```python
from build123d import *


with BuildPart() as part:
    # Sketch1 → Base-Revolve (revolve)
    with BuildSketch(Plane.XY, mode=Mode.PRIVATE) as base_revolve_sk:
        with BuildLine():
            Line((0, 8), (0, 6.794144144))
            ThreePointArc((0, 6.794144144), (0.796034843, 5.848666431), (-0.1025, 5))
            Line((-0.1025, 5), (-40.113248654, 5))
            Line((-40.113248654, 5), (-43, 10))
            Line((-43, 10), (-43, 0))
            Line((-43, 0), (-5.783270352, 0))
            Line((-5.783270352, 0), (-3.5, 3.8))
            Line((-3.5, 3.8), (0, 3.8))
            ThreePointArc((0, 3.8), (2, 5.9), (0, 8))
        make_face()
    revolve(base_revolve_sk.sketch.rotate(Axis((40.376928104, 0, 0), (-1, 0, 0)), 90), axis=Axis((40.376928104, 0, 0), (-1, 0, 0)))


solid = part.part
```
Geometry check sheet. Reference: the model listing, model coordinates, mm. A direction names the side the tool comes from. Round coordinates to 2 decimals unless told otherwise and drop trailing zeros. Order: outer loops, then holes, each group sorted by start corner. A loop starts at its lowest first (then second) coordinate and runs counter-clockwise, first axis right, second up. Notation, with made-up numbers: (82.5, 82) - (108.5, 82) arc R15 cw to (108.5, 90) - close; hole circle Ø5 at (56.25, 14). An arc over 180 degrees is marked (long way). Use a Markdown table: item, result. Add a question column.
(1) Material ranges on line 1 along Y through (x, z) = (-1.7, 0); line 2 along X through (y, z) = (5.5, 0.25); line 3 along X through (y, z) = (-3.75, -3.75), recorded low to high. Write a range as [from, to].
(2) Sectioned sample at A-A, the plane x = -25. Enter the section's corners in (y, z), and give its area (3 significant figures).
(3) Tool access check on faces 1 (the flat face through (-43, 0, 0)), 2 (the cylindrical face through (-1.726, -1.141, -3.625)), 3 (the conical face through (-40.294, -1.596, -5.067)). Record the directions out of +Z, -Z, +X, -X, +Y, -Y that give a thin tool (end or side, any length) a straight path to the whole face; none if there is none.
(4) Depth check by flat-ended pin: pin 1 (10 mm diameter, centred on x = -27, z = -5, fed in from -Y); pin 2 (8 mm diameter, centred on x = -5.5, z = -7.5, fed in from +Y); pin 3 (10 mm diameter, centred on x = -27, y = 0, fed in from -Z). Enter the tip coordinate at first touch or a pass-through.
(5) Release check for a two-part mould opening along Z. For faces 4 (the flat face through (0, 6, 4)), 5 (the cylindrical face through (-20, 0, 5)), 6 (the conical face through (-5.387, -0.198, -0.629)) record: pulls with the +Z half, pulls with the -Z half, needs draft (parallel to the pull), parting line crosses it, or undercut.
Answers below:
| question | item | result |
|---|---|---|
| 1 | line 1 | [-5, -3.8], [3.8, 5] |
| 1 | line 2 | [-43, -40.41], [0.71, 1.96] |
| 1 | line 3 | [-43, -40.29], [0.57, 1.91] |
| 2 | outline | circle Ø10 at (0, 0) |
| 2 | area | 78.5 mm² |
| 3 | face 1 | +Z, -Z, -X, +Y, -Y |
| 3 | face 2 | +X |
| 3 | face 3 | none |
| 4 | pin 1 | y = -5 |
| 4 | pin 2 | y = 3.57 |
| 4 | pin 3 | z = -5 |
| 5 | face 4 | needs draft |
| 5 | face 5 | parting line crosses it |
| 5 | face 6 | undercut |
